```python
from build123d import *

# Parameters (mm, degrees)
EXTRUDE_1_DEPTH = 8
EXTRUDE_2_DEPTH = 10


with BuildPart() as part:
    # Эскиз1 → Повернуть1 (revolve)
    with BuildSketch(Plane.XY, mode=Mode.PRIVATE) as revolve_1_sk:
        Polygon((0, 0), (-28, 0), (-28, 2), (-30, 2), (-30, 8), (-15, 20), (-6, 20), (-6, 28), (-6, 76.4), (-4.4, 78), (0, 78), align=None)
    revolve(revolve_1_sk.sketch.rotate(Axis((0, 0, 0), (0, 1, 0)), 180), axis=Axis((0, 0, 0), (0, 1, 0)))  # turned: the seam where the file's is

    # Эскиз2 → Бобышка-Вытянуть1 (add)
    with BuildSketch(Plane(origin=(0, 20, 0), x_dir=(1, 0, 0), z_dir=(0, 1, 0))):
        Polygon((0, 10.969655115), (-9.5, 5.484827557), (-9.5, -5.484827557), (0, -10.969655115), (9.5, -5.484827557), (9.5, 5.484827557), align=None)
    extrude(amount=EXTRUDE_1_DEPTH)

    # Эскиз3 → Бобышка-Вытянуть2 (add)
    with BuildSketch(Plane(origin=(0, 52.2, 0), x_dir=(1, 0, 0), z_dir=(0, 1, 0))):
        Polygon((9.5, 5.484827557), (0, 10.969655115), (-9.5, 5.484827557), (-9.5, -5.484827557), (0, -10.969655115), (9.5, -5.484827557), align=None)
    extrude(amount=EXTRUDE_2_DEPTH)

    # Эскиз4 → Вырез-Повернуть2 (revolve, cut)
    with BuildSketch(Plane.XY, mode=Mode.PRIVATE) as cut_revolve_2_sk:
        Polygon((-18.160254038, 62.2), (-9.5, 62.2), (-18.160254038, 57.2), align=None)
        Polygon((-18.160254038, 52.2), (-18.160254038, 57.2), (-9.5, 52.2), align=None)
        Polygon((-16.42820323, 28), (-16.42820323, 24), (-9.5, 28), align=None)
        Polygon((-16.42820323, 24), (-16.42820323, 20), (-9.5, 20), align=None)
    revolve(cut_revolve_2_sk.sketch.rotate(Axis((0, 78, 0), (0, 1, 0)), 180), axis=Axis((0, 78, 0), (0, 1, 0)), mode=Mode.SUBTRACT)  # turned: the seam where the file's is


solid = part.part
```
Source: CAD feature listing. Evaluate the final solid. Frame: model axes, mm. A direction names the side the tool comes from. Give positions to 0.01 mm unless a question says otherwise; leave off trailing zeros. Write each loop counter-clockwise with the first axis right and the second up, starting at its lowest first coordinate (ties: lowest second). Pieces come first, ordered by that corner, then holes.
1. Section query A-A (y = 6). Return the cut outline in (x, z), then the cut area to 3 significant figures.
2. Access query for faces 1 (the face through (5.723, 39.931, -1.802)), 2 (the face through (4.684, 23.944, 8.266)), 3 (the face through (-0.02, 27.8, 9.85)), 4 (the face through (5.723, 69.201, -1.802)). Directions: +Z, -Z, +X, -X, +Y, -Y. A direction counts if a zero-diameter tool reaches every point of the face in a straight line with its end or side. Return the directions, or none.
3. Material intervals for line 1 along Y through (x, z) = (6, 9); line 2 along Z through (x, y) = (-5.5, 56); line 3 along Z through (x, y) = (2.5, 23.5), sorted ascending.
4. Section query C-C (y = 32). Return the cut outline in (x, z).
5. Pull-direction query (Y, two-part tool) for faces 5 (the face through (-9.5, 57, 0)), 6 (the face through (0.02, 52.4, -9.85)), 7 (the face through (-0.1, 62.2, 6.2)); classes: +Y half, -Y half, draft (parallel to the pull), parting line (faces both ways), or undercut.
6. First-contact query: pin 1 (3 mm diameter, centred on y = 18, z = -12, fed in from +X); pin 2 (6.5 mm diameter, centred on y = 23.5, z = -1.5, fed in from -X); pin 3 (10 mm diameter, centred on x = 4.5, z = 13.5, fed in from +Y); pin 4 (1 mm diameter, centred on y = 29, z = -8, fed in from +X). Flat tips, straight axial feed; report the tip coordinate or a pass-through.
7. Section query B-B (y = 55). Return the cut outline in (x, z), then the cut area to 3 significant figures.
Output values:
1. outline: circle Ø60 at (0, 0)
1. area: 2,830 mm2
2. face 1: none
2. face 2: +Z, +X, +Y
2. face 3: +Z
2. face 4: +Y
3. line 1: y = 0 to 20
3. line 2: z = -7.79 to 7.79
3. line 3: z = -9.53 to 9.53
4. outline: circle Ø12 at (0, 0)
5. face 5: draft
5. face 6: undercut
5. face 7: +Y half
6. pin 1: stops at x = 15.47
6. pin 2: stops at x = -9.5
6. pin 3: stops at y = 62.2
6. pin 4: passes through
7. outline: (-9.5, -5.48) - (0, -10.97) - (9.5, -5.48) - (9.5, 5.48) - (0, 10.97) - (-9.5, 5.48) - close
7. area: 313 mm2
